from build123d import *

# Parameters (mm, degrees)
F0_W     = 300
F0_H     = 232.072148
F1_DEPTH = 25
F2_R     = 7.605799
F3_DEPTH = 50
F4_R     = 65.713133
F5_DEPTH = 50


with BuildPart() as f1:
    # F0 (on Front) → F1 (new body)
    with BuildSketch(Plane.XZ):
        with Locations((-9.545375, -11.807603)):
            Rectangle(F0_W, F0_H)
    extrude(amount=F1_DEPTH)

    # F2 (on face) → F3 (join, symmetric)
    with BuildSketch(Plane.XZ.offset(25)):
        with Locations((-23.156079, -6.691449)):
            Circle(F2_R)
    extrude(amount=F3_DEPTH, both=True)

    # F4 (on face) → F5 (join, symmetric)
    with BuildSketch(Plane.XZ.offset(25)):
        with Locations((56.600176, -1.484662)):
            Circle(F4_R)
    extrude(amount=F5_DEPTH, both=True)


solid = f1.part
CAD build for the part. Positions are in the model's coordinates, mm. A direction names the side the tool comes from. Round coordinates to 2 decimals unless told otherwise and drop trailing zeros. Write each loop counter-clockwise with the first axis right and the second up, starting at its lowest first coordinate (ties: lowest second). Pieces come first, ordered by that corner, then holes.
(1) Drop flat-ended pins along their axis: P1, Ø12, axis at x = 66, y = 10, coming from the +Z side; P2, Ø5, axis at x = -57.5, z = -100.5, coming from the +Y side; P3, Ø6, axis at x = -85, z = -2, coming from the -Y side; P4, Ø5, axis at x = -13, y = -33, coming from the -Z side. Give the stop position or say it passes through.
(2) Probe line 1 along Y through (x, z) = (-23, 10.5); line 2 along X through (y, z) = (-64, -10.5); line 3 along Z through (x, y) = (72, 9). List the from-to ranges inside material, lowest first.
(3) 3-axis set-ups, long thin cutter, end or side, ignore diameter. For faces 4 (the face through (56, -75, -1)), 5 (the face through (-30.755, -50.35, -6.357)), 6 (the face through (4.45, 12.33, -41.47)): which of +Z, -Z, +X, -X, +Y, -Y reach the whole face in a straight line?
(4) Slice it at C-C, the plane y = -30. Write the cut outline in (x, z).
(5) Slice it at B-B, the plane z = 6. Write the cut outline in (x, y).
(6) Slice it at A-A, the plane x = 103.5. Write the cut outline in (y, z).
(7) Slice it at D-D, the plane z = -80. Write the cut outline in (x, y).
(8) Mould opens along X. For faces 1 (the face through (-23, 25, -7)), 2 (the face through (140.455, -12, -13)), 3 (the face through (-30.755, 12.325, -6.357)) say: pulls with the +X half, pulls with the -X half, needs draft (parallel to the pull), parting line crosses it, or undercut.
From the geometry:
1. P1: stops at z = 64.14
1. P2: stops at y = 0
1. P3: stops at y = -25
1. P4: passes through
2. line 1: y = -25 to 0
2. line 2: x = -29.74 to -16.57, -8.49 to 121.69
2. line 3: z = -65.37 to 62.4
3. face 4: +Z, -Z, +X, -X, -Y
3. face 5: -Y
3. face 6: +Y
4. outline: circle Ø15.21 at (-23.16, -6.69); circle Ø131.43 at (56.6, -1.48)
5. outline: (-159.55, -25) - (-8.69, -25) - (-8.69, -75) - (121.89, -75) - (121.89, -25) - (140.45, -25) - (140.45, 0) - (121.89, 0) - (121.89, 25) - (-8.69, 25) - (-8.69, 0) - (-159.55, 0) - close
6. outline: (-75, -47.51) - (-25, -47.51) - (-25, -127.84) - (0, -127.84) - (0, -47.51) - (25, -47.51) - (25, 44.54) - (0, 44.54) - (0, 104.23) - (-25, 104.23) - (-25, 44.54) - (-75, 44.54) - close
7. outline: (-159.55, -25) - (140.45, -25) - (140.45, 0) - (-159.55, 0) - close
8. face 1: needs draft
8. face 2: pulls with the +X half
8. face 3: undercut
